from build123d import *

# Parameters (mm, degrees)
BOSS_EXTRUDE2_DEPTH = 2.38125


with BuildPart() as part:
    # Sketch1 → Boss-Extrude2 (new body)
    with BuildSketch(Plane(origin=(0, 0, 0), x_dir=(1, 0, 0), z_dir=(0, 1, 0))):
        Polygon((0, 73.66), (81.915, 73.66), (81.915, 64.788475447), (85.217, 64.788475447), (85.217, 57.612975447), (81.915, 57.612975447), (81.915, 51.040725447), (75.311, 51.040725447), (75.311, 53.072725447), (72.771, 53.072725447), (72.771, 51.040725447), (65.151, 51.040725447), (65.151, 48.246725447), (72.809250882, 48.246725447), (72.809250882, 46.214725447), (75.349250882, 46.214725447), (75.349250882, 48.246725447), (81.953250882, 48.246725447), (81.953250882, 41.674475447), (85.255250882, 41.674475447), (85.255250882, 34.498975447), (81.953250882, 34.498975447), (81.953250882, 28.281019423), (75.349250882, 28.281019423), (75.349250882, 30.313019423), (72.809250882, 30.313019423), (72.809250882, 28.281019423), (65.189250882, 28.281019423), (65.189250882, 26.884019423), (65.189250882, 25.487019423), (72.847501763, 25.487019423), (72.847501763, 23.455019423), (75.387501763, 23.455019423), (75.387501763, 25.487019423), (81.991501763, 25.487019423), (81.991501763, 18.560475447), (85.293501763, 18.560475447), (85.293501763, 11.384975447), (81.991501763, 11.384975447), (81.915, 0), (0, 0), (0, 11.384975447), (-3.302, 11.384975447), (-3.302, 18.560475447), (0.003462387, 18.560475447), (0.003462387, 25.132725447), (6.610924774, 25.132725447), (6.610924774, 23.455019423), (9.150924774, 23.455019423), (9.150924774, 25.487019423), (16.770924774, 25.487019423), (16.770924774, 28.281019423), (9.150924774, 28.281019423), (9.150924774, 30.313019423), (6.607462387, 30.313019423), (6.607462387, 27.926725447), (0.003462387, 27.926725447), (0.003462387, 34.498975447), (-3.302, 34.498975447), (-3.302, 38.016561862), (-3.302, 41.674475447), (0, 41.674475447), (0, 48.246725447), (6.604, 48.246725447), (6.604, 46.214725447), (9.144, 46.214725447), (9.144, 48.246725447), (16.764, 48.246725447), (16.764, 51.040725447), (9.144, 51.040725447), (9.144, 53.072725447), (6.604, 53.072725447), (6.604, 51.040725447), (0, 51.040725447), (0, 57.612975447), (-3.302, 57.612975447), (-3.302, 64.788475447), (0, 64.788475447), align=None)
    extrude(amount=-BOSS_EXTRUDE2_DEPTH)


solid = part.part
CAD build for the part. Positions are in the model's coordinates, mm. A direction names the side the tool comes from. Coordinates: 2 decimals unless noted, no trailing zeros. Loops run counter-clockwise (first coordinate to the right, second up) from the corner with the lowest first, then second, coordinate; pieces in that order, holes last. Notation, with made-up numbers: (48, 82.5) - (72, 82.5) arc R9 cw to (72, 88.5) - close; hole circle Ø1 at (-15.5, 65.5). An arc over 180 degrees is marked (long way). Use one line per item in the form item = value. Start each with the question number.
1) Flat gauge pins, fed straight in: pin 1 (1 mm diameter, centred on y = -1, z = -47.5, fed in from -X); pin 2 (10 mm diameter, centred on x = 29, z = -47.5, fed in from +Y); pin 3 (1.2 mm diameter, centred on x = 84.5, y = -2, fed in from -Z). Where does each tip first touch, or does it go through?
2) Band-saw the part on A-A (x = 5). Give the cut face in (y, z), and give its area (3 significant figures).
3) Two-plate mould, pull along Z, no slides. Class faces 4 (the face through (3, -1, -25.133)), 5 (the face through (81.915, -1, -69)), 6 (the face through (84, -1, -11.385)): +Z half, -Z half, draft (parallel to the pull), parting line (faces both ways), or undercut.
4) Band-saw the part on B-B (z = -32). Give the cut face in (x, y), and give its area (3 significant figures).
5) Drill centre lines: L1, parallel to Z at x = 13, y = -0.85; L2, parallel to Z at x = 1, y = -2.15; L3, parallel to X at y = -2, z = -5.5. Where is each one in solid material? Low to high. Write a range as from..to.
6) Tool access for faces 1 (the face through (81.992, -1, -22)), 2 (the face through (-2, -1, -57.613)), 3 (the face through (-2, -1, -64.788)): list every direction of +Z, -Z, +X, -X, +Y, -Y with a clear straight run to the whole face (end or side of a thin tool).
Check values:
q1.pin_1 = 0
q1.pin_2 = 0
q1.pin_3 = -64.79
q2.outline = (-2.38, -73.66) - (0, -73.66) - (0, -51.04) - (-2.38, -51.04) - close; (-2.38, -48.25) - (0, -48.25) - (0, -27.93) - (-2.38, -27.93) - close; (-2.38, -25.13) - (0, -25.13) - (0, 0) - (-2.38, 0) - close
q2.area = 162 mm2
q3.face_4 = undercut
q3.face_5 = draft
q3.face_6 = +Z half
q4.outline = (0, -2.38) - (81.95, -2.38) - (81.95, 0) - (0, 0) - close
q4.area = 195 mm2
q5.L1 = -73.66..-51.04, -48.25..-28.28, -25.49..0
q5.L2 = -73.66..-51.04, -48.25..-27.93, -25.13..0
q5.L3 = 0..81.95
q6.face_1 = +X, +Y, -Y
q6.face_2 = -X, +Y, -Y
q6.face_3 = -Z, -X, +Y, -Y
